from build123d import *

# Parameters (mm, degrees)
F0_W     = 50.8
F0_H     = 50.8
F1_DEPTH = 25.4
F2_R     = 5
F3_R     = 5
F4_R     = 15
F5_DEPTH = 25.4


with BuildPart() as f1:
    # F0 (on Front) → F1 (new body)
    with BuildSketch(Plane.XZ):
        with Locations((-25.4, 25.4)):
            Rectangle(F0_W, F0_H)
    extrude(amount=F1_DEPTH)

    # F2
    f2_edges = [f1.edges().sort_by_distance(p)[0] for p in [
        (-50.8, -12.7, 50.8),
    ]]
    fillet(f2_edges, radius=F2_R)

    # F3
    f3_edges = [f1.edges().sort_by_distance(p)[0] for p in [
        (0, -12.7, 50.8),
    ]]
    fillet(f3_edges, radius=F3_R)

    # F4 (on face) → F5 (cut, through all)
    with BuildSketch(Plane.XZ.offset(25.4)):
        with Locations((-25.188129, 25.400884)):
            Circle(F4_R)
    extrude(amount=-F5_DEPTH, mode=Mode.SUBTRACT)


solid = f1.part
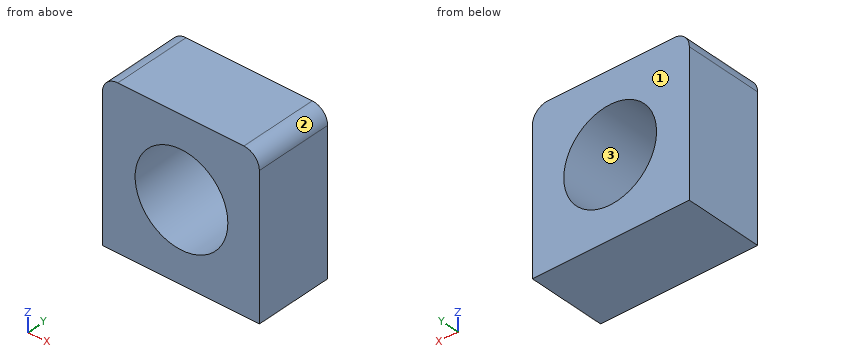
Here's how the part is built. I have some questions about the finished solid (model axes, mm). Face numbers are marked on the shaded views. Round coordinates to 2 decimals unless told otherwise and drop trailing zeros. Loops run counter-clockwise (first coordinate to the right, second up) from the corner with the lowest first, then second, coordinate; pieces in that order, holes last. Notation, with made-up numbers: (6.5, -30) - (60.5, -30) arc R11 ccw to (60.5, -22) - close; hole circle Ø11 at (-28.75, -16.75). An arc over 180 degrees is marked (long way). One line per question, with ' | ' between items. Start each with the question number.
Q1. I want a section at A-A (x = -28.5). Write out the boundary of the cut face in (y, z).
Q2. I want a section at C-C (y = -12.75). Write out the boundary of the cut face in (x, z).
Q3. I want a section at B-B (z = 28.5). Write out the boundary of the cut face in (x, y), then the cut area to 3 significant figures.
Q4. Please list where these lines run through material, in increasing order: line 1 (X direction, y = -9.25, z = 32.5); line 2 (X direction, y = -18.5, z = 30); line 3 (Z direction, x = -14, y = -7.25). Write a range as [from, to].
Q5. We'd pull the mould along Z, two halves only. Please class the marked faces 1, 2 and 3: +Z half, -Z half, draft (parallel to the pull), parting line (faces both ways), or undercut.
Response values:
1) outline: (-25.4, 0) - (0, 0) - (0, 10.77) - (-25.4, 10.77) - close; (-25.4, 40.03) - (0, 40.03) - (0, 50.8) - (-25.4, 50.8) - close
2) outline: (-50.8, 0) - (0, 0) - (0, 45.8) arc R5 ccw to (-5, 50.8) - (-45.8, 50.8) arc R5 ccw to (-50.8, 45.8) - close; hole circle Ø30 at (-25.19, 25.4)
3) outline: (-50.8, -25.4) - (-39.86, -25.4) - (-39.86, 0) - (-50.8, 0) - close; (-10.51, -25.4) - (0, -25.4) - (0, 0) - (-10.51, 0) - close | area: 545 mm²
4) line 1: x = [-50.8, -38.4], [-11.97, 0] | line 2: x = [-50.8, -39.47], [-10.91, 0] | line 3: z = [0, 15.41], [35.39, 50.8]
5) face 1: draft | face 2: +Z half | face 3: undercut
